Autodesk Inventor part; units mm, degrees
ref_plane "YZ Plane" through (0, 0, 0) normal (1, 0, 0) x (0, 1, 0)
ref_plane "XZ Plane" through (0, 0, 0) normal (0, 1, 0) x (-1, 0, 0)
ref_plane "XY Plane" through (0, 0, 0) normal (0, 0, 1) x (1, 0, 0)
sketch "Sketch1" plane through (0, 0, 0) normal (0, 0, 1) x (1, 0, 0)
  circle A0 centre (0, 4) radius 2
  circle A1 centre (-4, 0) radius 2
  circle A2 centre (0, -4) radius 2
  circle A3 centre (4, 0) radius 2
  line L0 (7, 40) -> (-7, 40)
  line L1 (8, 11.7321) -> (15.5744, 40)
  line L2 (7, 8) -> (40.1288, 8) construction
  line L3 (15.5744, 40) -> (7, 40)
  line L4 (-8, 11.7321) -> (-15.5744, 40)
  line L5 (-15.5744, 40) -> (-7, 40)
  line L6 (8, 0) -> (8, 11.7321)
  line L7 (-8, 0) -> (-8, 11.7321)
  arc A4 (-8, 0) -> (8, 0) centre (0, 0) ccw
  dimension "d2" = 4
  dimension "d5" = 360
extrude "Extrusion1" add sketch "Sketch1" along normal blind 5
sketch "Sketch2" plane through (0, 0, 0) normal (0, 0, -1) x (-1, 0, 0)
  circle A0 centre (0, 0) radius 6.625
  dimension "d18" = 13.25
extrude "Extrusion2" cut sketch "Sketch2" against normal blind 2
sketch "Sketch3" plane through (0, 0, 0) normal (0, 0, -1) x (-1, 0, 0)
  line L0 (-8, 11.7321) -> (-15.5744, 40)
  line L1 (-15.5744, 40) -> (15.5744, 40)
  line L2 (-15.5744, 40) -> (15.5744, 40)
  line L3 (15.5744, 40) -> (14.5391, 36.1363)
  line L4 (15.5744, 40) -> (8, 11.7321)
  line L5 (14.5391, 36.1363) -> (-14.5391, 36.1363)
  line L6 (-14.5391, 36.1363) -> (-15.5744, 40)
  point P0 (0, 0)
  dimension "d21" = 4
extrude "Extrusion3" add sketch "Sketch3" along normal blind 73.5
properties part number "OutPut_Shaft_From_Gearbox"
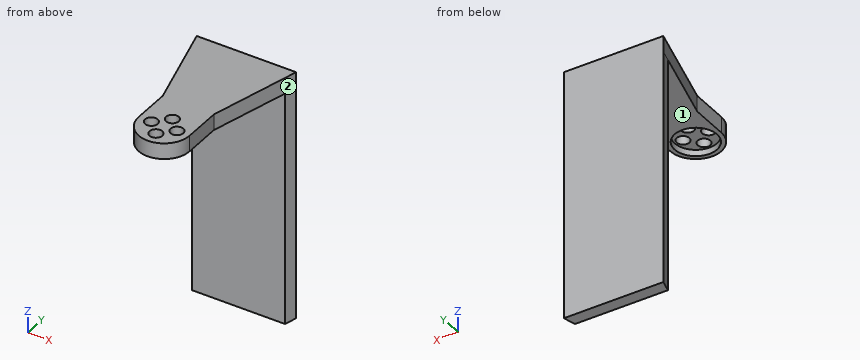
Check sheet for the modelled part. Datum: model origin and axes. Units: mm. Face numbers are marked on the shaded views. A direction names the side the tool comes from. Give positions to 0.01 mm unless a question says otherwise; leave off trailing zeros. Write each loop counter-clockwise with the first axis right and the second up, starting at its lowest first coordinate (ties: lowest second). Pieces come first, ordered by that corner, then holes.
Item 1: Cross-section at D-D (y = 10). Enter the section's corners in (x, z).
Item 2: Access from +Z, -Z, +X, -X, +Y, -Y to the whole of each face (thin tool, end or side, straight path). Record for the marked faces 1 and 2.
Item 3: Gauge pin test, flat ends, axial feed: pin 1 (2.5 mm diameter, centred on y = 4, z = 1.5, fed in from +X); pin 2 (8.5 mm diameter, centred on x = -1.5, z = -38.5, fed in from -Y); pin 3 (14.5 mm diameter, centred on x = 2.5, y = 22.5, fed in from -Z); pin 4 (3 mm diameter, centred on x = 0, y = 4, fed in from +Z). Record the tip position at first contact, or that the pin passes through.
Item 4: Scan lines: L1, parallel to X at y = 0, z = 4; L2, parallel to Y at x = 0, z = 2.7; L3, parallel to X at y = 4, z = 3.7. Record each from-to range of solid material in increasing order.
Item 5: Cross-section at B-B (y = 4). Enter the section's corners in (x, z), and give its area (3 significant figures).
Item 6: Cross-section at A-A (x = 0). Enter the section's corners in (y, z) (3 decimals).
Item 7: Cross-section at C-C (x = 4). Enter the section's corners in (y, z).
Report:
1. outline: (-8, 0) - (8, 0) - (8, 5) - (-8, 5) - close
2. face 1: -Z, +X, -X, -Y
2. face 2: +Z, -Z, +X, -Y
3. pin 1: stops at x = 8
3. pin 2: stops at y = 36.14
3. pin 3: stops at z = 0
3. pin 4: passes through
4. L1: x = -8 to -6, -2 to 2, 6 to 8
4. L2: y = -8 to -6, -2 to 2, 6 to 40
4. L3: x = -8 to -2, 2 to 8
5. outline: (-8, 0) - (-5.28, 0) - (-5.28, 2) - (-2, 2) - (-2, 5) - (-8, 5) - close; (2, 2) - (5.28, 2) - (5.28, 0) - (8, 0) - (8, 5) - (2, 5) - close
5. area: 46.9 mm2
6. outline: (-8, 0) - (-6.625, 0) - (-6.625, 2) - (-6, 2) - (-6, 5) - (-8, 5) - close; (-2, 2) - (2, 2) - (2, 5) - (-2, 5) - close; (6, 2) - (6.625, 2) - (6.625, 0) - (36.136, 0) - (36.136, -73.5) - (40, -73.5) - (40, 5) - (6, 5) - close
7. outline: (-6.93, 0) - (-5.28, 0) - (-5.28, 2) - (-2, 2) - (-2, 5) - (-6.93, 5) - close; (2, 2) - (5.28, 2) - (5.28, 0) - (36.14, 0) - (36.14, -73.5) - (40, -73.5) - (40, 5) - (2, 5) - close
